```python
from build123d import *

# Parameters (mm, degrees)
CYLINDER028_R     = 2
CYLINDER028_DEPTH = 10
CYLINDER029_R     = 2
CYLINDER029_DEPTH = 10
CYLINDER030_R     = 2
CYLINDER030_DEPTH = 10
CYLINDER031_R     = 2
CYLINDER031_DEPTH = 10
BOX014_W          = 20
BOX014_H          = 4
BOX014_DEPTH      = 1.5
CHAMFER002_SIZE   = 1
BOX013_W          = 178
BOX013_H          = 11
BOX013_DEPTH      = 12
BOX011_W          = 1.8
BOX011_H          = 98
BOX011_DEPTH      = 12
BOX012_W          = 1.8
BOX012_H          = 98
BOX012_DEPTH      = 12
BOX005_W          = 178
BOX005_H          = 192
BOX005_DEPTH      = 3


with BuildPart() as cilindro007:
    # Cylinder028 → Cylinder028 (new body)
    with BuildSketch(Plane(origin=(20, 144, 0), x_dir=(1, 0, 0), z_dir=(0, 0, 1))):
        Circle(CYLINDER028_R)
    extrude(amount=CYLINDER028_DEPTH)


with BuildPart() as cilindro008:
    # Cylinder029 → Cylinder029 (new body)
    with BuildSketch(Plane(origin=(160, -36, 0), x_dir=(1, 0, 0), z_dir=(0, 0, 1))):
        Circle(CYLINDER029_R)
    extrude(amount=CYLINDER029_DEPTH)


with BuildPart() as cilindro009:
    # Cylinder030 → Cylinder030 (new body)
    with BuildSketch(Plane(origin=(20, -36, 0), x_dir=(1, 0, 0), z_dir=(0, 0, 1))):
        Circle(CYLINDER030_R)
    extrude(amount=CYLINDER030_DEPTH)


with BuildPart() as cilindro010:
    # Cylinder031 → Cylinder031 (new body)
    with BuildSketch(Plane(origin=(160, 144, 0), x_dir=(1, 0, 0), z_dir=(0, 0, 1))):
        Circle(CYLINDER031_R)
    extrude(amount=CYLINDER031_DEPTH)


with BuildPart() as chamfer002:
    # Box014 → Box014 (new body)
    with BuildSketch(Plane(origin=(76, -34.2, 3), x_dir=(1, 0, 0), z_dir=(0, 0, 1))):
        with Locations((10, 2)):
            Rectangle(BOX014_W, BOX014_H)
    extrude(amount=BOX014_DEPTH)

    # Chamfer002
    chamfer002_edges = [chamfer002.edges().sort_by_distance(p)[0] for p in [
        (76, -34.2, 3.75),
        (96, -34.2, 3.75),
    ]]
    chamfer(chamfer002_edges, length=CHAMFER002_SIZE)


with BuildPart() as cubo009:
    # Box013 → Box013 (new body)
    with BuildSketch(Plane(origin=(1, 90, 3), x_dir=(1, 0, 0), z_dir=(0, 0, 1))):
        with Locations((89, 5.5)):
            Rectangle(BOX013_W, BOX013_H)
    extrude(amount=BOX013_DEPTH)


with BuildPart() as fusion011:
    # Box011 → Box011 (new body)
    with BuildSketch(Plane(origin=(1, 0, 3), x_dir=(1, 0, 0), z_dir=(0, 0, 1))):
        with Locations((0.9, 49)):
            Rectangle(BOX011_W, BOX011_H)
    extrude(amount=BOX011_DEPTH)

    # Fusion011: union Cubo009
    add(cubo009.part)


with BuildPart() as fusion012:
    # Box012 → Box012 (new body)
    with BuildSketch(Plane(origin=(177.2, 0, 3), x_dir=(1, 0, 0), z_dir=(0, 0, 1))):
        with Locations((0.9, 49)):
            Rectangle(BOX012_W, BOX012_H)
    extrude(amount=BOX012_DEPTH)

    # Fusion012: union Fusion011
    add(fusion011.part)


with BuildPart() as cut049:
    # Box005 → Box005 (new body)
    with BuildSketch(Plane(origin=(1, -45, 0), x_dir=(1, 0, 0), z_dir=(0, 0, 1))):
        with Locations((89, 96)):
            Rectangle(BOX005_W, BOX005_H)
    extrude(amount=BOX005_DEPTH)

    # Fusion013: union Fusion012
    add(fusion012.part)

    # Fusion014: union Chamfer002
    add(chamfer002.part)

    # Cut046: cut Cilindro010
    add(cilindro010.part, mode=Mode.SUBTRACT)

    # Cut047: cut Cilindro009
    add(cilindro009.part, mode=Mode.SUBTRACT)

    # Cut048: cut Cilindro008
    add(cilindro008.part, mode=Mode.SUBTRACT)

    # Cut049: cut Cilindro007
    add(cilindro007.part, mode=Mode.SUBTRACT)


solid = cut049.part
```
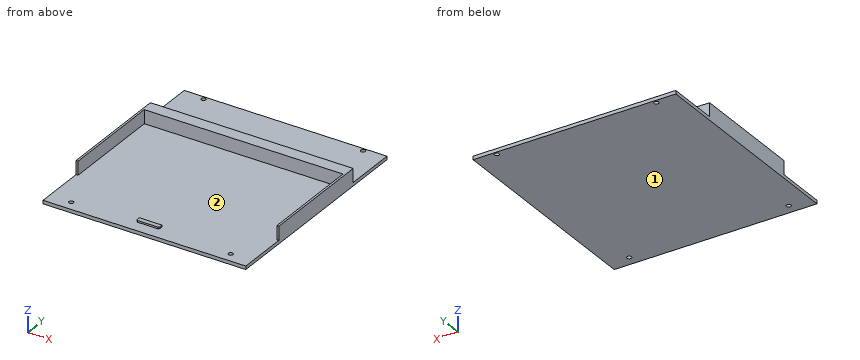
Part model, mm, in its own coordinate system. Face numbers are marked on the shaded views. Coordinates: 2 decimals unless noted, no trailing zeros. Order: outer loops, then holes, each group sorted by start corner. A loop starts at its lowest first (then second) coordinate and runs counter-clockwise, first axis right, second up. Notation, with made-up numbers: (89.5, 52.25) -> (139.5, 52.25) arc R19 cw to (139.5, 58.25) -> close; hole circle Ø11 at (-18.75, 27). An arc over 180 degrees is marked (long way). Put each result on its own line as item: value. Start each with the question number.
(1) Mould opens along X. For the marked faces 1 and 2 say: pulls with the +X half, pulls with the -X half, needs draft (parallel to the pull), parting line crosses it, or undercut.
(2) Probe line 1 along X through (y, z) = (-36, 2.1); line 2 along Y through (x, z) = (20, 2.05); line 3 along X through (y, z) = (78.5, 8). List the from-to ranges inside material, lowest first. Write a range as [from, to].
(3) Pin check, flat tips, straight feed: pin 1 Ø4.5 at (x, y) = (86, -31.5) entering from +Z; pin 2 Ø1 at (x, y) = (145, 39.5) entering from -Z; pin 3 Ø0.9 at (x, z) = (2.5, 12) entering from -Y; pin 4 Ø1 at (x, y) = (77, 2) entering from +Z. Stop position of each tip, or through.
(4) Band-saw the part on A-A (y = 70.5). Give the cut face in (x, z).
(5) Band-saw the part on C-C (y = -22.5). Give the cut face in (x, z), then the cut area to 3 significant figures.
(6) Band-saw the part on B-B (z = 9.25). Give the cut face in (x, y).
Determined:
1. face 1: needs draft
1. face 2: undercut
2. line 1: x = [1, 18], [22, 158], [162, 179]
2. line 2: y = [-45, -38], [-34, 142], [146, 147]
2. line 3: x = [1, 2.8], [177.2, 179]
3. pin 1: stops at z = 4.5
3. pin 2: stops at z = 0
3. pin 3: stops at y = 0
3. pin 4: stops at z = 3
4. outline: (1, 0) -> (179, 0) -> (179, 15) -> (177.2, 15) -> (177.2, 3) -> (2.8, 3) -> (2.8, 15) -> (1, 15) -> close
5. outline: (1, 0) -> (179, 0) -> (179, 3) -> (1, 3) -> close
5. area: 534 mm²
6. outline: (1, 0) -> (2.8, 0) -> (2.8, 90) -> (177.2, 90) -> (177.2, 0) -> (179, 0) -> (179, 101) -> (1, 101) -> close
